The listing builds one solid part. Answer for the finished solid, in the listing's coordinates (mm). A direction names the side the tool comes from. Coordinates: 2 decimals unless noted, no trailing zeros. Loops run counter-clockwise (first coordinate to the right, second up) from the corner with the lowest first, then second, coordinate; pieces in that order, holes last. Notation, with made-up numbers: (21, 80) - (75, 80) arc R27 ccw to (75, 111) - close; hole circle Ø3 at (28.25, 58.25). An arc over 180 degrees is marked (long way). One line per question, with ' | ' between items.
Autodesk Inventor part; units mm, degrees
ref_plane "YZ Plane" through (0, 0, 0) normal (1, 0, 0) x (0, 1, 0)
ref_plane "XZ Plane" through (0, 0, 0) normal (0, 1, 0) x (-1, 0, 0)
ref_plane "XY Plane" through (0, 0, 0) normal (0, 0, 1) x (1, 0, 0)
sketch "Sketch1" plane through (0, 0, 0) normal (0, 0, 1) x (1, 0, 0)
  circle A0 centre (0, 0) radius 25
  dimension "d0" = 50
extrude "Extrusion1" add sketch "Sketch1" along normal blind 3
sketch "Sketch2" plane through (0, 0, 3) normal (0, 0, 1) x (1, 0, 0)
  circle A0 centre (0, 0) radius 5
  dimension "d3" = 10
extrude "Extrusion2" add sketch "Sketch2" along normal blind 5
sketch "Sketch3" plane through (0, 0, 8) normal (0, 0, 1) x (1, 0, 0)
  circle A0 centre (0, 0) radius 2.5
  dimension "d6" = 5
extrude "Extrusion3" cut sketch "Sketch3" against normal blind 5
sketch "Sketch4" plane through (0, 0, 0) normal (0, 1, 0) x (-1, 0, 0)
  point P0 (0, 0)
sketch "Sketch5" plane through (0, 0, 0) normal (0, 1, 0) x (-1, 0, 0)
  point P0 (0, 0)
sketch "Sketch6" plane through (0, 0, 0) normal (0, 1, 0) x (-1, 0, 0)
  point P0 (0, 0)
sketch "Sketch7" plane through (0, 0, 0) normal (0, 1, 0) x (-1, 0, 0)
  line L0 (5, 8) -> (-5, 8)
  line L1 (0, 8) -> (0, 3)
  line L2 (25, 3) -> (-25, 3)
  circle A0 centre (0, 5.5) radius 1.25
  point P0 (0, 0)
  dimension "d9" = 2.5
extrude "Extrusion4" cut sketch "Sketch7" along normal blind 6.1125
thread "Thread1"
properties part number "Tampa_RoloA"
Item 1: Find section C-C, the plane z = 1.25. Write down the section's boundary in (x, y), plus the area to 3 significant figures.
Taken from the geometry:
outline: circle Ø50 at (0, 0) | area: 1,960 mm2
Item 2: Find section A-A, the plane x = 0. Write down the section's boundary in (y, z), plus the area to 3 significant figures.
Taken from the geometry:
outline: (-25, 0) - (25, 0) - (25, 3) - (5, 3) - (5, 4.25) - (2.5, 4.25) - (2.5, 3) - (-2.5, 3) - (-2.5, 8) - (-5, 8) - (-5, 3) - (-25, 3) - close; (2.5, 6.75) - (5, 6.75) - (5, 8) - (2.5, 8) - close | area: 169 mm2
Item 3: Find section D-D, the plane x = 12. Write down the section's boundary in (y, z), plus the area to 3 significant figures.
Taken from the geometry:
outline: (-21.93, 0) - (21.93, 0) - (21.93, 3) - (-21.93, 3) - close | area: 132 mm2
Item 4: Find section B-B, the plane y = 0. Write down the section's boundary in (x, z).
Taken from the geometry:
outline: (-25, 0) - (25, 0) - (25, 3) - (5, 3) - (5, 8) - (2.5, 8) - (2.5, 3) - (-2.5, 3) - (-2.5, 8) - (-5, 8) - (-5, 3) - (-25, 3) - close
Item 5: Which of the six approach directions +Z, -Z, +X, -X, +Y, -Y give full straight-line access (tool end or side, diameter ignored) to faces 1 (the face through (0, 0, 0)), 2 (the face through (0, 0, 3))?
Taken from the geometry:
face 1: -Z, +X, -X, +Y, -Y | face 2: +Z
Item 6: The mould has two halves that part along X. Classify faces 3 (the face through (2, -2, 8)), 4 (the face through (0.27, 3.56, 6.72)), 5 (the face through (23.846, -7.509, 1.479)), 6 (the face through (-0.54, -2.44, 5.54)): pulls with the +X half, pulls with the -X half, needs draft (parallel to the pull), parting line crosses it, or undercut.
Taken from the geometry:
face 3: needs draft | face 4: undercut | face 5: parting line crosses it | face 6: undercut
Item 7: Find the intervals of material crossed by line 1 (Z direction, x = 0, y = 3.15); line 2 (Y direction, x = 0, z = 5.75); line 3 (Y direction, x = 0, z = 4.05), in increasing order. Write a range as [from, to].
Taken from the geometry:
line 1: z = [0, 4.25], [6.75, 8] | line 2: y = [-5, -2.5] | line 3: y = [-5, -2.5], [2.5, 5]
Item 8: Each of these flat-tipped pins is pushed along its axis until it touches: pin 1 Ø1.5 at (x, z) = (0, 5.5) entering from -Y; pin 2 Ø4.5 at (x, y) = (0, 0) entering from +Z; pin 3 Ø1 at (x, z) = (13.5, 2) entering from +Y. Where does it stop, or does it pass through?
Taken from the geometry:
pin 1: stops at y = -5 | pin 2: stops at z = 3 | pin 3: stops at y = 21.35
